```python
from build123d import *

# Parameters (mm, degrees)
EXTRUDE_1_DEPTH     = 22
CUT_EXTRUDE_1_REACH = 136.239
SKETCH_2_W          = 15
SKETCH_2_H          = 11
SKETCH_3_R          = 26
CUT_EXTRUDE_2_DEPTH = 12
CUT_EXTRUDE_3_REACH = 125.806
SKETCH_4_R          = 17.5
SKETCH_5_R          = 23.5
CUT_EXTRUDE_4_DEPTH = 7
CHAMFER_1_SIZE      = 1
CUT_EXTRUDE_5_REACH = 127.172
SKETCH_6_R          = 2.75
CUT_EXTRUDE_7_REACH = 127.172
CUT_EXTRUDE_8_DEPTH = 4


with BuildPart() as part:
    # 草图1 → 凸台-拉伸1 (new body)
    with BuildSketch(Plane(origin=(0, 0, 0), x_dir=(1, 0, 0), z_dir=(0, 1, 0))):
        with BuildLine():
            Line((0, 28), (-120, 28))
            Line((-120, 28), (-120, -28))
            Line((-120, -28), (0, -28))
            ThreePointArc((0, -28), (28, 0), (0, 28))
        make_face()
    extrude(amount=EXTRUDE_1_DEPTH)

    # 草图2 → 切除-拉伸1 (cut, up to next)
    with BuildSketch(Plane.XY.offset(28), mode=Mode.PRIVATE) as cut_extrude_1_sk1:
        with Locations((-112.5, 5.5)):
            Rectangle(SKETCH_2_W, SKETCH_2_H)
    cut_extrude_1_tool1 = extrude(cut_extrude_1_sk1.sketch, amount=-CUT_EXTRUDE_1_REACH, mode=Mode.PRIVATE) & part.part
    add(cut_extrude_1_tool1.solids().sort_by_distance((-112.5, 5.5, 28))[0], mode=Mode.SUBTRACT)

    # 草图3 → 切除-拉伸2 (cut)
    with BuildSketch(Plane(origin=(0, 22, 0), x_dir=(1, 0, 0), z_dir=(0, 1, 0))):
        with Locations(Location((0, 0, 0), (0, 0, 270))):
            Circle(SKETCH_3_R)
    extrude(amount=-CUT_EXTRUDE_2_DEPTH, mode=Mode.SUBTRACT)

    # 草图4 → 切除-拉伸3 (cut, up to next)
    with BuildSketch(Plane(origin=(0, 10, 0), x_dir=(1, 0, 0), z_dir=(0, 1, 0)), mode=Mode.PRIVATE) as cut_extrude_3_sk1:
        with Locations(Location((0, 0, 0), (0, 0, 270))):
            Circle(SKETCH_4_R)
    cut_extrude_3_tool1 = extrude(cut_extrude_3_sk1.sketch, amount=-CUT_EXTRUDE_3_REACH, mode=Mode.PRIVATE) & part.part
    add(cut_extrude_3_tool1.solids().sort_by_distance((0, 10, 0))[0], mode=Mode.SUBTRACT)

    # 草图5 → 切除-拉伸4 (cut)
    with BuildSketch(Plane.XZ):
        with Locations(Location((0, 0, 0), (0, 0, 270))):
            Circle(SKETCH_5_R)
    extrude(amount=-CUT_EXTRUDE_4_DEPTH, mode=Mode.SUBTRACT)

    # 倒角1
    chamfer_1_edges = [part.edges().sort_by_distance(p)[0] for p in [
        (0, 22, -26),
        (0, 10, -17.5),
        (0, 0, 23.5),
        (0, 7, -17.5),
    ]]
    chamfer(chamfer_1_edges, length=CHAMFER_1_SIZE)

    # 草图6 → 切除-拉伸5 (cut, up to next)
    with BuildSketch(Plane(origin=(0, 22, 0), x_dir=(1, 0, 0), z_dir=(0, 1, 0)), mode=Mode.PRIVATE) as cut_extrude_5_sk1:
        with Locations(Location((-112.5, 0, 0), (0, 0, 270))):
            Circle(SKETCH_6_R)
    cut_extrude_5_tool1 = extrude(cut_extrude_5_sk1.sketch, amount=-CUT_EXTRUDE_5_REACH, mode=Mode.PRIVATE) & part.part
    # 草图6 → 切除-拉伸5 (cut, up to next)
    with BuildSketch(Plane(origin=(0, 22, 0), x_dir=(1, 0, 0), z_dir=(0, 1, 0)), mode=Mode.PRIVATE) as cut_extrude_5_sk2:
        with Locations(Location((-112.5, 16, 0), (0, 0, 270))):
            Circle(SKETCH_6_R)
    cut_extrude_5_tool2 = extrude(cut_extrude_5_sk2.sketch, amount=-CUT_EXTRUDE_5_REACH, mode=Mode.PRIVATE) & part.part
    # 草图6 → 切除-拉伸5 (cut, up to next)
    with BuildSketch(Plane(origin=(0, 22, 0), x_dir=(1, 0, 0), z_dir=(0, 1, 0)), mode=Mode.PRIVATE) as cut_extrude_5_sk3:
        with Locations(Location((-112.5, -16, 0), (0, 0, 270))):
            Circle(SKETCH_6_R)
    cut_extrude_5_tool3 = extrude(cut_extrude_5_sk3.sketch, amount=-CUT_EXTRUDE_5_REACH, mode=Mode.PRIVATE) & part.part
    add(cut_extrude_5_tool1.solids().sort_by_distance((-112.5, 22, 0))[0], mode=Mode.SUBTRACT)
    add(cut_extrude_5_tool2.solids().sort_by_distance((-112.5, 22, -16))[0], mode=Mode.SUBTRACT)
    add(cut_extrude_5_tool3.solids().sort_by_distance((-112.5, 22, 16))[0], mode=Mode.SUBTRACT)

    # 草图8 → 切除-拉伸7 (cut, up to next)
    with BuildSketch(Plane(origin=(0, 22, 0), x_dir=(1, 0, 0), z_dir=(0, 1, 0)), mode=Mode.PRIVATE) as cut_extrude_7_sk1:
        with BuildLine():
            ThreePointArc((-42.5, -13), (-39.5, -16), (-42.5, -19))
            Line((-42.5, -19), (-92.5, -19))
            ThreePointArc((-92.5, -19), (-95.5, -16), (-92.5, -13))
            Line((-92.5, -13), (-42.5, -13))
        make_face()
    cut_extrude_7_tool1 = extrude(cut_extrude_7_sk1.sketch, amount=-CUT_EXTRUDE_7_REACH, mode=Mode.PRIVATE) & part.part
    add(cut_extrude_7_tool1.solids().sort_by_distance((-67.5, 22, 16))[0], mode=Mode.SUBTRACT)

    # 草图8<3> → 切除-拉伸8 (cut)
    with BuildSketch(Plane(origin=(0, 22, 0), x_dir=(1, 0, 0), z_dir=(0, 1, 0))):
        Polygon((-92.5, -12), (-42.5, -12), (-40.191634991, -12.001796941), (-37.883271378, -16), (-40.191636387, -19.998205479), (-42.5, -20), (-92.5, -20), (-94.808363613, -19.998205479), (-97.116728622, -16), (-94.808365009, -12.001796941), align=None)
    extrude(amount=-CUT_EXTRUDE_8_DEPTH, mode=Mode.SUBTRACT)


solid = part.part
```
The listing builds one solid part. Answer for the finished solid, in the listing's coordinates (mm). A direction names the side the tool comes from. Coordinates: 2 decimals unless noted, no trailing zeros. Loops run counter-clockwise (first coordinate to the right, second up) from the corner with the lowest first, then second, coordinate; pieces in that order, holes last. Notation, with made-up numbers: (81, 81.25) - (95, 81.25) arc R25 ccw to (95, 94.25) - close; hole circle Ø5 at (86.5, 2). An arc over 180 degrees is marked (long way). Use a Markdown table: item, result. Add a question column.
1) The mould has two halves that part along Z. Classify faces 1 (the flat face through (-109, 11, 0)), 2 (the cylindrical face through (-15.821, 15.577, -20.633)), 3 (the cylindrical face through (27.993, 10.846, 0.616)): released by +Z, released by -Z, zero draft, split by the parting line, or undercut.
2) Find the intervals of material crossed by line 1 (X direction, y = 15, z = 0); line 2 (Z direction, x = -88, y = 15.75); line 3 (X direction, y = 17, z = 1), in increasing order.
3) Given pin 1 (23.5 mm diameter, centred on x = -3.5, z = 7, fed in from -Y); pin 2 (5 mm diameter, centred on x = 7.5, y = 14.5, fed in from +Z); pin 3 (15.5 mm diameter, centred on x = -3, z = 12.5, fed in from +Y); pin 4 (4.5 mm diameter, centred on x = -112.5, z = 16, fed in from -Y), each flat-ended and moving along its own axis, determine where each tip first touches the part or whether it passes through.
4) The part is cut by section A-A, the plane z = 0. State how many separate pieces and enclosed holes the cut face has, and give its area (3 significant figures).
5) For faces 4 (the flat face through (-95.98, 20.03, 14.03)), 5 (the flat face through (-105, 5, 0)), 6 (the flat face through (-68, 9, 13)), determine the directions among +Z, -Z, +X, -X, +Y, -Y from which every point of the face is accessible in a straight line to the end or side of a thin tool.
6) The part is cut by section C-C, the plane y = 14. Give the vertices of the cut face in (x, z).
7) The part is cut by section D-D, the plane x = -79. Give the vertices of the cut face in (y, z).
8) The part is cut by section B-B, the plane x = -112.5. Give the vertices of the cut face in (y, z), and give its area (4 significant figures).
Here are the results:
| question | item | result |
|---|---|---|
| 1 | face 1 | zero draft |
| 1 | face 2 | undercut |
| 1 | face 3 | split by the parting line |
| 2 | line 1 | x = -120 to -115.25, -109.75 to -26, 26 to 28 |
| 2 | line 2 | z = -28 to 13, 19 to 28 |
| 2 | line 3 | x = -120 to -115.06, -109.94 to -25.98, 25.98 to 27.98 |
| 3 | pin 1 | stops at y = 7 |
| 3 | pin 2 | stops at z = 27.55 |
| 3 | pin 3 | stops at y = 10 |
| 3 | pin 4 | passes through |
| 4 | separate pieces | 3 |
| 4 | enclosed holes | 0 |
| 4 | area | 1,970 mm^2 |
| 5 | face 4 | +Y |
| 5 | face 5 | +Z, -Z, -X, -Y |
| 5 | face 6 | +Y, -Y |
| 6 | outline | (-120, -28) - (0, -28) arc R28 ccw to (0, 28) - (-120, 28) - close; hole circle Ø5.5 at (-112.5, -16); hole circle Ø5.5 at (-112.5, 0); hole circle Ø5.5 at (-112.5, 16); hole (-92.5, 13) - (-42.5, 13) arc R3 ccw to (-42.5, 19) - (-92.5, 19) arc R3 ccw to start; hole circle Ø52 at (0, 0) |
| 7 | outline | (0, -28) - (22, -28) - (22, 12) - (18, 12) - (18, 13) - (0, 13) - close; (0, 19) - (18, 19) - (18, 20) - (22, 20) - (22, 28) - (0, 28) - close |
| 8 | outline | (11, -28) - (22, -28) - (22, -18.75) - (11, -18.75) - close; (11, -13.25) - (22, -13.25) - (22, -2.75) - (11, -2.75) - close; (11, 2.75) - (22, 2.75) - (22, 13.25) - (11, 13.25) - close; (11, 18.75) - (22, 18.75) - (22, 28) - (11, 28) - close |
| 8 | area | 434.5 mm^2 |
